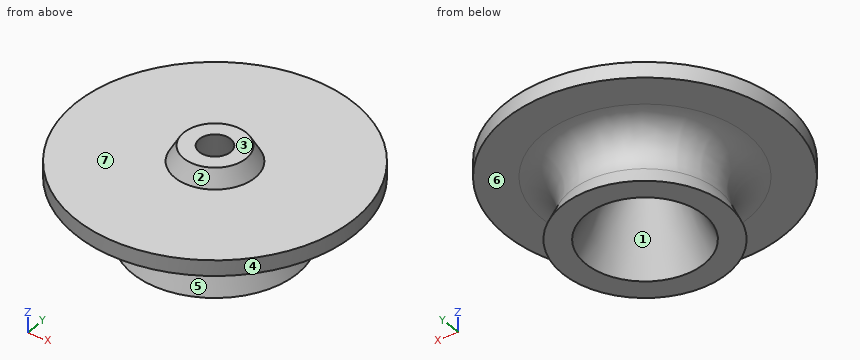
from build123d import *

# Parameters (mm, degrees)
FILLET1_R = 12.7


with BuildPart() as part:
    # Sketch1 → Revolve1 (revolve)
    with BuildSketch(Plane(origin=(0, 0, 0), x_dir=(1, 0, 0), z_dir=(0, 1, 0))):
        Polygon((-6.402170304, -5.603691702), (-24.16849208, 32.496308298), (-33.69349208, 32.496308298), (-21.849277563, 7.096308298), (-57.003438355, 7.096308298), (-57.003438355, 0.746308298), (-16.369673719, 0.746308298), (-12.752170304, -5.603691702), align=None)
    revolve(axis=Axis((0, 0, -42.597586509), (0, 0, 1)))

    # Fillet1
    fillet1_edges = [part.edges().sort_by_distance(p)[0] for p in [
        (21.849277563, 0, -7.096308298),
    ]]
    fillet(fillet1_edges, radius=FILLET1_R)


solid = part.part
Input: part model. Units: mm. Frame: model coordinates. Face numbers are marked on the shaded views. A direction names the side the tool comes from. Round coordinates to 2 decimals unless told otherwise and drop trailing zeros. Loops run counter-clockwise (first coordinate to the right, second up) from the corner with the lowest first, then second, coordinate; pieces in that order, holes last. Notation, with made-up numbers: (17, -38) -> (65, -38) arc R10 ccw to (65, -19) -> close; hole circle Ø8 at (-34.5, 73.5). An arc over 180 degrees is marked (long way). Answer as a JSON object with one key per item and string values. Group by question number.
1) Draft query along Y for the marked faces 1, 2 and 3. Return one class per face: +Y half, -Y half, draft (parallel to the pull), parting line (faces both ways), or undercut.
2) Pin query (flat end, axial travel): pin 1 (3 mm diameter, centred on y = -38.5, z = -5.5, fed in from -X); pin 2 (8 mm diameter, centred on x = 36, z = -13.5, fed in from -Y); pin 3 (10 mm diameter, centred on x = -12.5, z = -19, fed in from +Y); pin 4 (8 mm diameter, centred on x = -26.5, z = -10.5, fed in from +Y). Return the tip coordinate at first contact, or that it passes through.
3) Reachability of the marked faces 4, 5, 6 and 7 from +Z, -Z, +X, -X, +Y, -Y: full face, straight path, thin tool, end or side. Return the list, or none.
4) Ray query, L1, parallel to Z at x = -10, y = -42.5; L2, parallel to Y at x = -11, z = -29; L3, parallel to X at y = -6.5, z = -8.5. Return the intervals inside material, ascending.
5) Section query D-D on x = 47. Output: boundary loops of the cut face in (y, z).
6) Section query A-A on x = 0. Output: boundary loops of the cut face in (y, z).
7) Section query C-C on z = -30. Output: boundary loops of the cut face in (x, y), plus the area to 3 significant figures.
Reply:
{
 "1": {"face 1": "undercut", "face 2": "parting line", "face 3": "draft"},
 "2": {"pin 1": "stops at x = -43.36", "pin 2": "passes through", "pin 3": "stops at y = 28.48", "pin 4": "stops at y = 51.52"},
 "3": {"face 4": "+Z, -Z", "face 5": "none", "face 6": "-Z", "face 7": "+Z"},
 "4": {"L1": "z = -7.1 to -0.75", "L2": "y = -30.12 to -19.67, 19.67 to 30.12", "L3": "x = -35.39 to -11.23, 11.23 to 35.39"},
 "5": {"outline": "(-32.26, -7.1) -> (32.26, -7.1) -> (32.26, -0.75) -> (-32.26, -0.75) -> close"},
 "6": {"outline": "(-57, -7.1) -> (-41.78, -7.1) arc R12.7 cw to (-30.27, -25.16) -> (-33.69, -32.5) -> (-24.17, -32.5) -> (-6.4, 5.6) -> (-12.75, 5.6) -> (-16.37, -0.75) -> (-57, -0.75) -> close; (6.4, 5.6) -> (24.17, -32.5) -> (33.69, -32.5) -> (30.27, -25.16) arc R12.7 cw to (41.78, -7.1) -> (57, -7.1) -> (57, -0.75) -> (16.37, -0.75) -> (12.75, 5.6) -> close"},
 "7": {"outline": "circle Ø65.06 at (0, 0); hole circle Ø46.01 at (0, 0)", "area": "1,660 mm2"}
}
